Here's how the part is built. I have some questions about the finished solid (model axes, mm). Face numbers are marked on the shaded views. A direction names the side the tool comes from. Coordinates: 2 decimals unless noted, no trailing zeros. Order: outer loops, then holes, each group sorted by start corner. A loop starts at its lowest first (then second) coordinate and runs counter-clockwise, first axis right, second up. Notation, with made-up numbers: (-28.75, 52.25) - (17.25, 52.25) arc R9 ccw to (17.25, 62.25) - close; hole circle Ø2 at (31.25, 74). An arc over 180 degrees is marked (long way). Use one line per item in the form item = value. Start each with the question number.
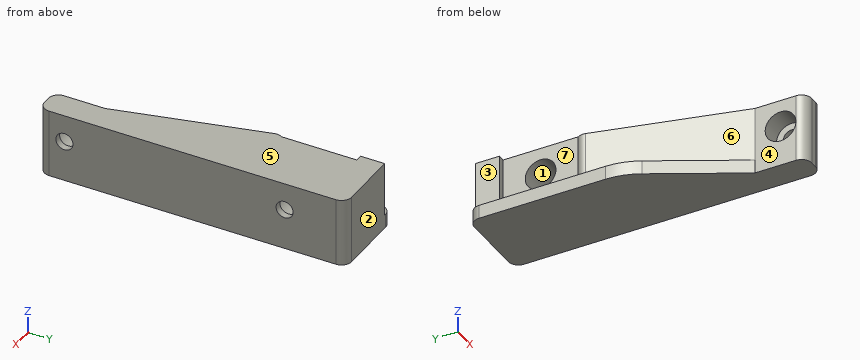
from build123d import *

# Parameters (mm, degrees)
SKETCH1_W            = 24
SKETCH1_H            = 90
BOSS_EXTRUDE1_DEPTH  = 20
CUT_EXTRUDE1_DEPTH   = 16
CUT_EXTRUDE8_DEPTH   = 10
SKETCH11_R           = 2.5
CUT_EXTRUDE9_DEPTH   = 18.5
SKETCH12_R           = 4.5
CUT_EXTRUDE10_DEPTH  = 16.5
FILLET1_R            = 20
FILLET2_R            = 3
FILLET1_OF_MIRROR1_R = 20
FILLET2_OF_MIRROR1_R = 3
SKETCH13_W           = 28.58864277
SKETCH13_H           = 106.823904202
CUT_EXTRUDE11_DEPTH  = 24


with BuildPart() as part:
    # Sketch1 → Boss-Extrude1 (new body)
    with BuildSketch(Plane.XY):
        with Locations((12, 45)):
            Rectangle(SKETCH1_W, SKETCH1_H)
    boss_extrude1 = extrude(amount=-BOSS_EXTRUDE1_DEPTH)

    # Sketch4 → Cut-Extrude1 (cut)
    with BuildSketch(Plane.XY):
        Polygon((20.5, 83), (18.5, 83), (18.5, 61), (19.5, 61), (8, 15), (8, 0), (24, 0), (24, 90), (20.5, 90), align=None)
    cut_extrude1 = extrude(amount=-CUT_EXTRUDE1_DEPTH, mode=Mode.SUBTRACT)

    # Sketch9 → Cut-Extrude8 (cut)
    with BuildSketch(Plane(origin=(0, 0, -20), x_dir=(-1, 0, 0), z_dir=(0, 0, -1))):
        Polygon((-24, 0), (-24, 45), (-8, 15), (-8, 0), align=None)
    cut_extrude8 = extrude(amount=-CUT_EXTRUDE8_DEPTH, mode=Mode.SUBTRACT)

    # Sketch11 → Cut-Extrude9 (cut)
    with BuildSketch(Plane(origin=(18.5, 0, 0), x_dir=(0, 0, -1), z_dir=(1, 0, 0))):
        with Locations(Location((8, 72, 0), (0, 0, 90))):
            Circle(SKETCH11_R)
        with Locations(Location((8, 7.5, 0), (0, 0, 90))):
            Circle(SKETCH11_R)
    cut_extrude9 = extrude(amount=-CUT_EXTRUDE9_DEPTH, mode=Mode.SUBTRACT)

    # Sketch12 → Cut-Extrude10 (cut)
    with BuildSketch(Plane(origin=(18.5, 0, 0), x_dir=(0, 0, -1), z_dir=(1, 0, 0))):
        with Locations(Location((8, 72, 0), (0, 0, 90))):
            Circle(SKETCH12_R)
        with Locations(Location((8, 7.5, 0), (0, 0, 90))):
            Circle(SKETCH12_R)
    cut_extrude10 = extrude(amount=-CUT_EXTRUDE10_DEPTH, mode=Mode.SUBTRACT)

    # Fillet1
    fillet1_edges = [part.edges().sort_by_distance(p)[0] for p in [
        (24, 45, -18),
    ]]
    fillet(fillet1_edges, radius=FILLET1_R)

    # Fillet2
    # the kernel refuses this fillet: 3 mm, written as the material it takes off along each edge
    with BuildSketch(Plane(origin=(0, 90, 7.5), x_dir=(1, 0, 0), z_dir=(0, 0, -1)), Plane(origin=(0, 0, 7.5), x_dir=(0, 1, 0), z_dir=(0, 0, -1)), Plane(origin=(8, 0, -27.5), x_dir=(0, 1, 0), z_dir=(0, 0, 1))) as fillet2_piece_1:
        with BuildLine():
            CenterArc((FILLET2_R, FILLET2_R), FILLET2_R, 180, 90)
            Line((0, FILLET2_R), (-FILLET2_R * 0.02, FILLET2_R))
            Line((-FILLET2_R * 0.02, FILLET2_R), (-FILLET2_R * 0.02, -FILLET2_R * 0.02))
            Line((-FILLET2_R * 0.02, -FILLET2_R * 0.02), (FILLET2_R, -FILLET2_R * 0.02))
            Line((FILLET2_R, -FILLET2_R * 0.02), (FILLET2_R, 0))
        make_face()
    extrude(amount=35, mode=Mode.SUBTRACT)
    with BuildSketch(Plane(origin=(24, 90, -8.5), x_dir=(0, -1, 0), z_dir=(0, 0, -1))) as fillet2_piece_2:
        with BuildLine():
            CenterArc((FILLET2_R, FILLET2_R), FILLET2_R, 180, 90)
            Line((0, FILLET2_R), (-FILLET2_R * 0.02, FILLET2_R))
            Line((-FILLET2_R * 0.02, FILLET2_R), (-FILLET2_R * 0.02, -FILLET2_R * 0.02))
            Line((-FILLET2_R * 0.02, -FILLET2_R * 0.02), (FILLET2_R, -FILLET2_R * 0.02))
            Line((FILLET2_R, -FILLET2_R * 0.02), (FILLET2_R, 0))
        make_face()
    extrude(amount=19, mode=Mode.SUBTRACT)
    with BuildSketch(Plane(origin=(19.5, 61, 6.128837665), x_dir=(-0.24253562503633366, -0.9701425001453317, 0), z_dir=(0, 0, -1))) as fillet2_piece_3:
        with BuildLine():
            CenterArc((2.451535066, 3), FILLET2_R, 222.580014358, 47.419985642)
            Line((0.242535625, 0.9701425), (0.198355636, 0.92954535))
            ThreePointArc((0.198355636, 0.92954535), (0.063059263, 0.499623388), (-0.05820855, 0.014552138))
            Line((-0.05820855, 0.014552138), (0, -0.06))
            Line((0, -0.06), (2.451535066, -0.06))
            Line((2.451535066, -0.06), (2.451535066, 0))
        make_face()
    extrude(amount=22.128837665, mode=Mode.SUBTRACT)


with BuildPart() as mirror1_1:
    # Mirror1: Boss-Extrude1 across plane
    add(boss_extrude1.mirror(Plane(origin=(24, 0, -20), x_dir=(0, 0, 1), z_dir=(1, 0, 0))))

    # Mirror1 2: Cut-Extrude1, Cut-Extrude8, Cut-Extrude9, Cut-Extrude10 across plane
    add(cut_extrude1.mirror(Plane(origin=(24, 0, -20), x_dir=(0, 0, 1), z_dir=(1, 0, 0))), mode=Mode.SUBTRACT)
    add(cut_extrude8.mirror(Plane(origin=(24, 0, -20), x_dir=(0, 0, 1), z_dir=(1, 0, 0))), mode=Mode.SUBTRACT)
    add(cut_extrude9.mirror(Plane(origin=(24, 0, -20), x_dir=(0, 0, 1), z_dir=(1, 0, 0))), mode=Mode.SUBTRACT)
    add(cut_extrude10.mirror(Plane(origin=(24, 0, -20), x_dir=(0, 0, 1), z_dir=(1, 0, 0))), mode=Mode.SUBTRACT)

    # Fillet1 of Mirror1
    fillet1_of_mirror1_edges = [mirror1_1.edges().sort_by_distance(p)[0] for p in [
        (24, 45, -18),
    ]]
    fillet(fillet1_of_mirror1_edges, radius=FILLET1_OF_MIRROR1_R)

    # Fillet2 of Mirror1
    # the kernel refuses this fillet: 3 mm, written as the material it takes off along each edge
    with BuildSketch(Plane(origin=(48, 90, 7.5), x_dir=(-1, 0, 0), z_dir=(0, 0, -1)), Plane(origin=(48, 0, 7.5), x_dir=(0, 1, 0), z_dir=(0, 0, -1))) as fillet2_of_mirror1_piece_1:
        with BuildLine():
            CenterArc((FILLET2_OF_MIRROR1_R, -FILLET2_OF_MIRROR1_R), FILLET2_OF_MIRROR1_R, 90, 90)
            Line((0, -FILLET2_OF_MIRROR1_R), (-FILLET2_OF_MIRROR1_R * 0.02, -FILLET2_OF_MIRROR1_R))
            Line((-FILLET2_OF_MIRROR1_R * 0.02, -FILLET2_OF_MIRROR1_R), (-FILLET2_OF_MIRROR1_R * 0.02, FILLET2_OF_MIRROR1_R * 0.02))
            Line((-FILLET2_OF_MIRROR1_R * 0.02, FILLET2_OF_MIRROR1_R * 0.02), (FILLET2_OF_MIRROR1_R, FILLET2_OF_MIRROR1_R * 0.02))
            Line((FILLET2_OF_MIRROR1_R, FILLET2_OF_MIRROR1_R * 0.02), (FILLET2_OF_MIRROR1_R, 0))
        make_face()
    extrude(amount=35, mode=Mode.SUBTRACT)
    with BuildSketch(Plane(origin=(24, 90, -8.5), x_dir=(0, -1, 0), z_dir=(0, 0, -1))) as fillet2_of_mirror1_piece_2:
        with BuildLine():
            CenterArc((FILLET2_OF_MIRROR1_R, -FILLET2_OF_MIRROR1_R), FILLET2_OF_MIRROR1_R, 90, 90)
            Line((0, -FILLET2_OF_MIRROR1_R), (-FILLET2_OF_MIRROR1_R * 0.02, -FILLET2_OF_MIRROR1_R))
            Line((-FILLET2_OF_MIRROR1_R * 0.02, -FILLET2_OF_MIRROR1_R), (-FILLET2_OF_MIRROR1_R * 0.02, FILLET2_OF_MIRROR1_R * 0.02))
            Line((-FILLET2_OF_MIRROR1_R * 0.02, FILLET2_OF_MIRROR1_R * 0.02), (FILLET2_OF_MIRROR1_R, FILLET2_OF_MIRROR1_R * 0.02))
            Line((FILLET2_OF_MIRROR1_R, FILLET2_OF_MIRROR1_R * 0.02), (FILLET2_OF_MIRROR1_R, 0))
        make_face()
    extrude(amount=19, mode=Mode.SUBTRACT)
    with BuildSketch(Plane(origin=(40, 0, 7.5), x_dir=(0, 1, 0), z_dir=(0, 0, -1))) as fillet2_of_mirror1_piece_3:
        with BuildLine():
            CenterArc((FILLET2_OF_MIRROR1_R, FILLET2_OF_MIRROR1_R), FILLET2_OF_MIRROR1_R, 180, 90)
            Line((0, FILLET2_OF_MIRROR1_R), (-FILLET2_OF_MIRROR1_R * 0.02, FILLET2_OF_MIRROR1_R))
            Line((-FILLET2_OF_MIRROR1_R * 0.02, FILLET2_OF_MIRROR1_R), (-FILLET2_OF_MIRROR1_R * 0.02, -FILLET2_OF_MIRROR1_R * 0.02))
            Line((-FILLET2_OF_MIRROR1_R * 0.02, -FILLET2_OF_MIRROR1_R * 0.02), (FILLET2_OF_MIRROR1_R, -FILLET2_OF_MIRROR1_R * 0.02))
            Line((FILLET2_OF_MIRROR1_R, -FILLET2_OF_MIRROR1_R * 0.02), (FILLET2_OF_MIRROR1_R, 0))
        make_face()
    extrude(amount=35, mode=Mode.SUBTRACT)
    with BuildSketch(Plane(origin=(28.5, 61, 6.128837665), x_dir=(0.24253562503633366, -0.9701425001453317, 0), z_dir=(0, 0, -1))) as fillet2_of_mirror1_piece_4:
        with BuildLine():
            CenterArc((2.451535066, -3), FILLET2_OF_MIRROR1_R, 90, 47.419985642)
            Line((0.242535625, -0.9701425), (0.198355636, -0.92954535))
            ThreePointArc((0.198355636, -0.92954535), (0.063059263, -0.499623388), (-0.05820855, -0.014552138))
            Line((-0.05820855, -0.014552138), (0, 0.06))
            Line((0, 0.06), (2.451535066, 0.06))
            Line((2.451535066, 0.06), (2.451535066, 0))
        make_face()
    extrude(amount=22.128837665, mode=Mode.SUBTRACT)


with BuildPart() as part_1:
    add(part.part)

    # Mirror1 united with what the copies touc: union Mirror1_1
    add(mirror1_1.part)

    # Sketch13 → Cut-Extrude11 (cut)
    with BuildSketch(Plane.ZY):
        with Locations((-8.954074045, 49.790814809)):
            Rectangle(SKETCH13_W, SKETCH13_H)
    extrude(amount=-CUT_EXTRUDE11_DEPTH, mode=Mode.SUBTRACT)


solid = part_1.part
1) For pin 1 (2 mm diameter, centred on y = 85.5, z = -7, fed in from -X); pin 2 (10 mm diameter, centred on y = 8, z = -6.5, fed in from -X); pin 3 (8 mm diameter, centred on y = 25.5, z = -15, fed in from -X), each with a flat end and sliding along its axis, tell me the tip position at first contact or that it passes through.
2) Suppose I cut it at C-C, the plane x = 35.25. List the corners of the cut face in (y, z) for me.
3) I need wall thicknesses on probe 1 along Z at (x, y) = (37.75, 72); probe 2 along Z at (x, y) = (46.65, 72); probe 3 along Y at (x, z) = (47.65, -8). Which ranges of each line are inside material? Lowest first, please. Write a range as [from, to].
4) Suppose I cut it at D-D, the plane y = 19.5. List the corners of the cut face in (x, z) for me (3 decimals), then the cut area to 3 significant figures.
5) Suppose I cut it at A-A, the plane y = 72. List the corners of the cut face in (x, z) for me.
6) Which directions (+Z, -Z, +X, -X, +Y, -Y) give clear straight access to the entire face, cutting with the end or side of a thin tool? Please do the marked faces 4, 5, 6 and 7.
7) Suppose I cut it at B-B, the plane z = -15. List the corners of the cut face in (x, y) for me, then the cut area to 3 significant figures.
8) If we mould it in two halves opening along Y, with no side actions, what happens to the marked faces 1, 2 and 3? For each: pulls with the +Y half, pulls with the -Y half, needs draft (parallel to the pull), parting line crosses it, or undercut.
From the geometry:
q1.pin_1 = 27.5
q1.pin_2 = 40
q1.pin_3 = 32.33
q2.outline = (23.91, -20) - (90, -20) - (90, 0) - (34, 0) - (34, -16) - (23.91, -16) - close; hole circle Ø9 at (72, -8)
q3.probe_1 = [-20, -12.5], [-3.5, 0]
q3.probe_2 = [-20, -10.5], [-5.5, 0]
q3.probe_3 = [1.59, 5], [10, 69.5], [74.5, 88.41]
q4.outline = (37.6, -20) - (48, -20) - (48, 0) - (38.875, 0) - (38.875, -16) - (37.6, -16) - close
q4.area = 188 mm2
q5.outline = (24, -20) - (48, -20) - (48, -10.5) - (46, -10.5) - (46, -12.5) - (29.5, -12.5) - (29.5, -16) - (24, -16) - close; (29.5, -3.5) - (46, -3.5) - (46, -5.5) - (48, -5.5) - (48, 0) - (29.5, 0) - close
q6.face_4 = +Z, -Z, -X, -Y
q6.face_5 = +Z, +X, -X, +Y, -Y
q6.face_6 = +Z, -X, -Y
q6.face_7 = +Z, -X
q7.outline = (27.5, 83) - (29.5, 83) - (29.5, 61) arc R3 ccw to (29.09, 58.62) - (40, 15) - (40, 3) arc R3 ccw to (43, 0) - (45, 0) arc R3 ccw to (48, 3) - (48, 87) arc R3 ccw to (45, 90) - (27.5, 90) - close
q7.area = 1,300 mm2
q8.face_1 = undercut
q8.face_2 = pulls with the +Y half
q8.face_3 = needs draft
